Design review of the part built by this model. Coordinates are the model's own, in mm. A direction names the side the tool comes from. Coordinates: 2 decimals unless noted, no trailing zeros. Write each loop counter-clockwise with the first axis right and the second up, starting at its lowest first coordinate (ties: lowest second). Pieces come first, ordered by that corner, then holes.
Q1. Mouldability with a two-part tool opening along Z and no side actions: class faces 1 (the conical face through (24.955, 0.741, -6.564)), 2 (the cylindrical face through (11.013, -4.056, -53.848)), 3 (the cylindrical face through (49.848, 0.713, -28.392)) as pulls with the +Z half, pulls with the -Z half, needs draft (parallel to the pull), parting line crosses it, or undercut.
Q2. For probe 1 along Z at (x, y) = (25.3, -5.75); probe 2 along Z at (x, y) = (25, -3); probe 3 along X at (y, z) = (-3.75, -6.3), list the stretches that pass through material, from the lowest coordinate up.
Q3. Machinability: for faces 4 (the flat face through (25, -4, -1.4)), 5 (the cylindrical face through (25.84, -4.2, -50.94)), 6 (the cylindrical face through (39.548, -4.056, -2.113)), 7 (the flat face through (10.3, -4, -28)), which of the approach directions +Z, -Z, +X, -X, +Y, -Y give a long, thin tool a straight path to every point of the face, cutting with its end or side? Answer none if there is none.
Q4. Insertion check: pin 1 (10 mm diameter, centred on x = 12.5, z = 13, fed in from -Y); pin 2 (2.5 mm diameter, centred on y = -3, z = -39.5, fed in from -X); pin 3 (6.5 mm diameter, centred on y = -5, z = -16, fed in from +X). Each pin has a flat end and moves straight along its axis. Give the tip position at first contact, or say it passes through.
Q5. Take a section at D-D (y = 25.3). Give the boundary of the cut face in (x, z), and give its area (3 significant figures).
Q6. Take a section at C-C (x = 44.5). Give the boundary of the cut face in (y, z), and give its area (3 significant figures).
Q7. Take a section at B-B (z = -28.5). Give the boundary of the cut face in (x, y).
Q8. Take a section at A-A (y = 42). Give the boundary of the cut face in (x, z).
```python
from build123d import *

# Parameters (mm, degrees)
SKETCH2_W                       = 50.6
SKETCH2_H                       = 56
BOSS_EXTRUDE1_DEPTH             = 50.6
SKETCH3_W                       = 30
SKETCH3_H                       = 53.2
BOSS_EXTRUDE2_DEPTH             = 8
TAP_DRILL_FOR_M6X1_0_TAP1_D     = 5
TAP_DRILL_FOR_M6X1_0_TAP1_DEPTH = 7.5000104
TAP_DRILL_FOR_M6X1_0_TAP1_TIP   = 1.502151548
TAP_DRILL_FOR_1_4_20_TAP1_D     = 5.1054
TAP_DRILL_FOR_1_4_20_TAP1_DEPTH = 7.62
TAP_DRILL_FOR_1_4_20_TAP1_TIP   = 1.533816902
SKETCH11_R                      = 14.2875
BOSS_EXTRUDE3_DEPTH             = 25.4
FILLET1_R                       = 2.5


with BuildPart() as part:
    # Sketch2 → Boss-Extrude1 (new body)
    with BuildSketch(Plane(origin=(0, 0, 0), x_dir=(1, 0, 0), z_dir=(0, 1, 0))):
        with Locations((25.3, 28)):
            Rectangle(SKETCH2_W, SKETCH2_H)
    extrude(amount=BOSS_EXTRUDE1_DEPTH)

    # Sketch3 → Boss-Extrude2 (add)
    with BuildSketch(Plane.XZ):
        with Locations((25.3, -28)):
            Rectangle(SKETCH3_W, SKETCH3_H)
    extrude(amount=BOSS_EXTRUDE2_DEPTH)

    # Tap Drill for M6x1.0 Tap1
    with Locations(Plane.XZ.offset(8)):
        with Locations((25.3, -35.25), (25.3, -48.5), (25.3, -6.3)):
            Hole(TAP_DRILL_FOR_M6X1_0_TAP1_D / 2, depth=TAP_DRILL_FOR_M6X1_0_TAP1_DEPTH)
            with Locations((0, 0, -(TAP_DRILL_FOR_M6X1_0_TAP1_DEPTH + TAP_DRILL_FOR_M6X1_0_TAP1_TIP / 2))):  # 118° drill point
                Cone(0, TAP_DRILL_FOR_M6X1_0_TAP1_D / 2, TAP_DRILL_FOR_M6X1_0_TAP1_TIP, mode=Mode.SUBTRACT)

    # Tap Drill for 1/4-20 Tap1
    with Locations(Plane.XZ.offset(8)):
        with Locations((25.3, -22)):
            Hole(TAP_DRILL_FOR_1_4_20_TAP1_D / 2, depth=TAP_DRILL_FOR_1_4_20_TAP1_DEPTH)
            with Locations((0, 0, -(TAP_DRILL_FOR_1_4_20_TAP1_DEPTH + TAP_DRILL_FOR_1_4_20_TAP1_TIP / 2))):  # 118° drill point
                Cone(0, TAP_DRILL_FOR_1_4_20_TAP1_D / 2, TAP_DRILL_FOR_1_4_20_TAP1_TIP, mode=Mode.SUBTRACT)

    # Sketch11 → Boss-Extrude3 (add)
    with BuildSketch(Plane.XY):
        with Locations(Location((25.3, 25.3, 0), (0, 0, 180))):
            Circle(SKETCH11_R)
    extrude(amount=BOSS_EXTRUDE3_DEPTH)

    # Fillet1
    fillet1_edges = [part.edges().sort_by_distance(p)[0] for p in [
        (50.6, 50.6, -28),
        (25.3, 50.6, -56),
        (10.3, -4, -1.4),
        (10.3, -4, -54.6),
        (40.3, -4, -54.6),
        (40.3, -4, -1.4),
        (0, 50.6, -28),
        (50.6, 0, -28),
        (0, 0, -28),
        (25.3, 50.6, 0),
        (0, 25.3, -56),
        (50.6, 25.3, -56),
        (50.6, 25.3, 0),
        (0, 25.3, 0),
    ]]
    fillet(fillet1_edges, radius=FILLET1_R)


solid = part.part
```
Response:
1. face 1: undercut
1. face 2: pulls with the -Z half
1. face 3: needs draft
2. probe 1: z = -54.6 to -51, -46 to -37.75, -32.75 to -24.55, -19.45 to -8.8, -3.8 to -1.4
2. probe 2: z = -54.6 to -50.98, -46.02 to -37.73, -32.77 to -24.54, -19.46 to -8.78, -3.82 to -1.4
2. probe 3: x = 10.3 to 22.8, 27.8 to 40.3
3. face 4: +Z, +X, -X, -Y
3. face 5: -Y
3. face 6: +Z, +X, -Y
3. face 7: +Z, -Z, -X, -Y
4. pin 1: stops at y = 13.33
4. pin 2: stops at x = 10.3
4. pin 3: stops at x = 40.3
5. outline: (0, -53.5) arc R2.5 ccw to (2.5, -56) - (48.1, -56) arc R2.5 ccw to (50.6, -53.5) - (50.6, -2.5) arc R2.5 ccw to (48.1, 0) - (39.59, 0) - (39.59, 25.4) - (11.01, 25.4) - (11.01, 0) - (2.5, 0) arc R2.5 ccw to (0, -2.5) - close
5. area: 3,550 mm2
6. outline: (0, -56) - (48.1, -56) arc R2.5 ccw to (50.6, -53.5) - (50.6, -2.5) arc R2.5 ccw to (48.1, 0) - (0, 0) - close
6. area: 2,830 mm2
7. outline: (0, 2.5) arc R2.5 ccw to (2.5, 0) - (10.3, 0) - (10.3, -8) - (40.3, -8) - (40.3, 0) - (48.1, 0) arc R2.5 ccw to (50.6, 2.5) - (50.6, 48.1) arc R2.5 ccw to (48.1, 50.6) - (2.5, 50.6) arc R2.5 ccw to (0, 48.1) - close
8. outline: (0, -53.5) arc R2.5 ccw to (2.5, -56) - (48.1, -56) arc R2.5 ccw to (50.6, -53.5) - (50.6, -2.5) arc R2.5 ccw to (48.1, 0) - (2.5, 0) arc R2.5 ccw to (0, -2.5) - close
